The model under review builds one solid part; all positions refer to its coordinate system, in mm. A direction names the side the tool comes from. Give positions to 0.01 mm unless a question says otherwise; leave off trailing zeros. Write each loop counter-clockwise with the first axis right and the second up, starting at its lowest first coordinate (ties: lowest second). Pieces come first, ordered by that corner, then holes. Notation, with made-up numbers: (47, -2) - (74, -2) arc R12 cw to (74, 3) - close; hole circle Ø7 at (-26.75, 49). An arc over 180 degrees is marked (long way). Write item = value, one per line.
Autodesk Fusion 360 part; units mm, degrees
sketch "Sketch1" plane through (0, 0, 0) normal (0, 0, 1) x (1, 0, 0)
  line L0 (0, 0) -> (60, 0)
  line L1 (60, 0) -> (60, 60)
  line L2 (60, 60) -> (0, 60)
  line L3 (0, 60) -> (0, 0)
  line L4 (60, 60) -> (0, 0) construction
  line L5 (0, 60) -> (60, 0) construction
  line L6 (30, 30) -> (30, 60) construction
  line L7 (30, 30) -> (30, 0) construction
  line L8 (17.3, 60) -> (17.3, 0) construction
  line L9 (42.7, 60) -> (42.7, 0) construction
  line L10 (0, 7) -> (60, 7) construction
  line L11 (0, 53) -> (60, 53) construction
  circle A0 centre (17.3, 53) radius 3.5
  circle A1 centre (17.3, 7) radius 3.5
  circle A2 centre (42.7, 7) radius 3.5
  circle A3 centre (42.7, 53) radius 3.5
  line L12 (13.8, 53) -> (13.8, 7)
  line L13 (20.8, 7) -> (20.8, 53)
  line L14 (39.2, 53) -> (39.2, 7)
  line L15 (46.2, 7) -> (46.2, 53)
  dimension "d1" = 60
  dimension "d2" = 60
  dimension "d3" = 12.7
  dimension "d4" = 12.7
  dimension "d5" = 23
  dimension "d8" = 23
  dimension "d9" = 7
  dimension "d10" = 7
  dimension "d11" = 7
  dimension "d12" = 7
extrude "Extrude1" add sketch "Sketch1" along normal blind 35
1. Draft analysis for pull direction X (two halves, no side actions). For faces 3 (the flat face through (0, 30, 17)), 4 (the flat face through (39.2, 30, 17)), 5 (the flat face through (60, 30, 17)), 6 (the flat face through (30, 0, 17)), state which applies: +X half, -X half, draft (parallel to the pull), parting line (faces both ways), or undercut.
Findings below:
face_3 = -X half
face_4 = undercut
face_5 = +X half
face_6 = draft
2. Take a section at B-B on x = 17.3. Give the boundary of the cut face in (y, z), and give its area (3 significant figures).
Findings below:
outline = (0, 0) - (3.5, 0) - (3.5, 35) - (0, 35) - close; (56.5, 0) - (60, 0) - (60, 35) - (56.5, 35) - close
area = 245 mm²
3. Take a section at C-C on z = 4. Give the boundary of the cut face in (x, y), and give its area (3 significant figures).
Findings below:
outline = (0, 0) - (60, 0) - (60, 60) - (0, 60) - close; hole (13.8, 7) arc R3.5 ccw to (20.8, 7) - (20.8, 53) arc R3.5 ccw to (13.8, 53) - close; hole (39.2, 7) arc R3.5 ccw to (46.2, 7) - (46.2, 53) arc R3.5 ccw to (39.2, 53) - close
area = 2,880 mm²
4. For line 1 (X direction, y = 21, z = 32.5); line 2 (Y direction, x = 43, z = 31.5); line 3 (X direction, y = 6, z = 10.5), list the stretches that pass through material, from the lowest coordinate up. Write a range as from..to.
Findings below:
line_1 = 0..13.8, 20.8..39.2, 46.2..60
line_2 = 0..3.51, 56.49..60
line_3 = 0..13.95, 20.65..39.35, 46.05..60
5. Take a section at A-A on y = 44. Give the boundary of the cut face in (x, z).
Findings below:
outline = (0, 0) - (13.8, 0) - (13.8, 35) - (0, 35) - close; (20.8, 0) - (39.2, 0) - (39.2, 35) - (20.8, 35) - close; (46.2, 0) - (60, 0) - (60, 35) - (46.2, 35) - close
6. Machinability: for faces 1 (the flat face through (30, 30, 35)), 2 (the flat face through (20.8, 30, 17)), which of the approach directions +Z, -Z, +X, -X, +Y, -Y give a long, thin tool a straight path to every point of the face, cutting with its end or side? Answer none if there is none.
Findings below:
face_1 = +Z, +X, -X, +Y, -Y
face_2 = +Z, -Z
